from build123d import *

# Parameters (mm, degrees)
SKETCH3_R               = 7.493
CUT_EXTRUDE2_DEPTH      = 8.9375
CUT_EXTRUDE2_DEPTH_BACK = 8.9375
SKETCH4_R               = 11.1125
SKETCH4_R_2             = 26.924
BOSS_EXTRUDE1_DEPTH     = 15.875
BOSS_EXTRUDE2_START     = 22.225
SKETCH7_R               = 6.35
BOSS_EXTRUDE2_DEPTH     = 4.7625
SKETCH5_R               = 2.4257
CUT_EXTRUDE3_DEPTH      = 27.9875
CUT_EXTRUDE3_DEPTH_BACK = 16.8750001


with BuildPart() as part:
    # Sketch1 → Revolve1 (revolve)
    with BuildSketch(Plane(origin=(0, 0, 0), x_dir=(0, 0, -1), z_dir=(1, 0, 0))):
        with BuildLine():
            Line((-20.6375, 0), (-26.9875, 0))
            Line((-26.9875, 0), (-26.9875, 7.9375))
            Line((-26.9875, 7.9375), (-25.587155577, 7.9375))
            ThreePointArc((-25.587155577, 7.9375), (-23.1775, 5.6515), (-20.767844423, 7.9375))
            Line((-20.767844423, 7.9375), (-19.3675, 7.9375))
            Line((-19.3675, 7.9375), (-19.3675, 5.495734842))
            Line((-19.3675, 5.495734842), (-20.6375, 4.7625))
            Line((-20.6375, 4.7625), (-20.6375, 0))
        make_face()
    revolve(axis=Axis((0, 0, 0), (0, 1, 0)))

    # Mirror1: part across plane


with BuildPart() as part_1:
    add(part.part)
    add(part.part.mirror(Plane(origin=(0, 0, 20.6375), x_dir=(0, 0, 1), z_dir=(0, 1, 0))))

    # Sketch3 → Cut-Extrude2 (cut, two sides)
    with BuildSketch(Plane(origin=(0, 0, 0), x_dir=(1, 0, 0), z_dir=(0, 1, 0))) as cut_extrude2_sk:
        with Locations((12.7, 0)):
            Circle(SKETCH3_R)
    extrude(amount=CUT_EXTRUDE2_DEPTH, mode=Mode.SUBTRACT)
    extrude(cut_extrude2_sk.sketch, amount=-CUT_EXTRUDE2_DEPTH_BACK, mode=Mode.SUBTRACT)

    # Sketch4 → Boss-Extrude1 (add, through all)
    with BuildSketch(Plane(origin=(0, 7.9375, 0), x_dir=(1, 0, 0), z_dir=(0, 1, 0))):
        Polygon((28.575, 28.575), (-53.975, 28.575), (-53.975, -12.7), (-12.7, -53.975), (28.575, -53.975), align=None)
        with Locations((-36.890166373, 9.525)):
            Circle(SKETCH4_R, mode=Mode.SUBTRACT)
        with Locations((9.525, -36.890166373)):
            Circle(SKETCH4_R, mode=Mode.SUBTRACT)
        Circle(SKETCH4_R_2, mode=Mode.SUBTRACT)
    extrude(amount=-BOSS_EXTRUDE1_DEPTH)


with BuildPart() as body_2:
    # Sketch7 → Boss-Extrude2 (new body)
    with BuildSketch(Plane(origin=(0, 7.9375, 0), x_dir=(1, 0, 0), z_dir=(0, 1, 0)).offset(BOSS_EXTRUDE2_START)):
        Polygon((28.575, -53.975), (28.575, 28.575), (-53.975, 28.575), (-53.975, -12.7), (-12.7, -53.975), align=None)
        Circle(SKETCH7_R, mode=Mode.SUBTRACT)
    extrude(amount=BOSS_EXTRUDE2_DEPTH)


with BuildPart() as cut_extrude3_tool:
    # Sketch5 → Cut-Extrude3 (new body, two sides)
    with BuildSketch(Plane(origin=(0, 7.9375, 0), x_dir=(1, 0, 0), z_dir=(0, 1, 0))) as cut_extrude3_sk:
        with Locations((23.8125, 23.8125)):
            Circle(SKETCH5_R)
        with Locations((-49.2125, 23.8125)):
            Circle(SKETCH5_R)
        with Locations((-23.933885369, 23.8125)):
            Circle(SKETCH5_R)
        with Locations((-49.2125, -10.727307909)):
            Circle(SKETCH5_R)
        with Locations((23.8125, -23.933885369)):
            Circle(SKETCH5_R)
        with Locations((23.8125, -49.2125)):
            Circle(SKETCH5_R)
        with Locations((-10.727307909, -49.2125)):
            Circle(SKETCH5_R)
    extrude(amount=CUT_EXTRUDE3_DEPTH)
    extrude(cut_extrude3_sk.sketch, amount=-CUT_EXTRUDE3_DEPTH_BACK)


with BuildPart() as part_2:
    add(part_1.part)

    # Cut-Extrude3: cut by cut_extrude3_tool
    add(cut_extrude3_tool.part, mode=Mode.SUBTRACT)


with BuildPart() as body_2_1:
    add(body_2.part)

    # Cut-Extrude3: cut by cut_extrude3_tool
    add(cut_extrude3_tool.part, mode=Mode.SUBTRACT)


solid = part_2.part
Model file for the job. Use its own axes, mm. A direction names the side the tool comes from. Round coordinates to 2 decimals unless told otherwise and drop trailing zeros. Loops run counter-clockwise (first coordinate to the right, second up) from the corner with the lowest first, then second, coordinate; pieces in that order, holes last.
1. Drop a flat-ended pin along its axis: P1, Ø3, axis at x = 23.81, z = -23.81, coming from the -Y side. Give the stop position or say it passes through.
Check values:
P1: passes through
2. Band-saw the part on C-C, the plane x = 0. List the corners of the cut face in (y, z) (1 decimal).
Check values:
outline: (-7.9, -28.6) - (7.9, -28.6) - (7.9, -25.6) arc R2.4 cw to (7.9, -20.8) - (7.9, -19.4) - (5.5, -19.4) - (4.8, -20.6) - (-4.8, -20.6) - (-5.5, -19.4) - (-7.9, -19.4) - (-7.9, -20.8) arc R2.4 cw to (-7.9, -25.6) - close; (-7.9, 19.4) - (-5.5, 19.4) - (-4.8, 20.6) - (4.8, 20.6) - (5.5, 19.4) - (7.9, 19.4) - (7.9, 20.8) arc R2.4 cw to (7.9, 25.6) - (7.9, 31.2) - (-7.9, 31.2) - (-7.9, 25.6) arc R2.4 cw to (-7.9, 20.8) - close; (-7.9, 42.6) - (7.9, 42.6) - (7.9, 54) - (-7.9, 54) - close
3. Wall check: probe 1 along X at (y, z) = (-0.5, 0) (1 decimal); probe 2 along Z at (x, y) = (25.5, 0.5) (3 decimals); probe 3 along Z at (x, y) = (17.5, 0.5) (1 decimal). Give the ranges that are in metal, low to high.
Check values:
probe 1: x = -54 to -42.6, -31.2 to -20.6, 20.6 to 28.6
probe 2: z = -28.575 to -25.555, -22.07 to 22.191, 25.676 to 47.47, 50.955 to 53.975
probe 3: z = -28.6 to -10.9, 10.9 to 29.2, 44.6 to 54
4. Band-saw the part on D-D, the plane x = 22.5. Count the separate pieces of the cut face and the enclosed holes in it, and give its area (3 significant figures).
Check values:
separate pieces: 4
enclosed holes: 0
area: 1,020 mm2
5. Band-saw the part on A-A, the plane x = -29.5. List the corners of the cut face in (y, z) (1 decimal).
Check values:
outline: (-7.9, -28.6) - (7.9, -28.6) - (7.9, -17.8) - (-7.9, -17.8) - close; (-7.9, -1.2) - (7.9, -1.2) - (7.9, 37.2) - (-7.9, 37.2) - close
6. Mould opens along Y. For faces 1 (the cylindrical face through (-46.972, 0.111, 11.656)), 2 (the flat face through (-14, -7.938, 14)), 3 (the cylindrical face through (-20.147, -0.067, -4.474)) say: +Y half, -Y half, draft (parallel to the pull), parting line (faces both ways), or undercut.
Check values:
face 1: draft
face 2: -Y half
face 3: undercut
7. Tool access for faces 4 (the flat face through (-12, 0, -28.575)), 5 (the conical face through (-17.378, 5.368, 9.039)), 6 (the cylindrical face through (20.193, -6.458, 0.062)): list every direction of +Z, -Z, +X, -X, +Y, -Y with a clear straight run to the whole face (end or side of a thin tool).
Check values:
face 4: -Z, +X, -X, +Y, -Y
face 5: none
face 6: +Y, -Y
8. Band-saw the part on B-B, the plane z = 0. List the corners of the cut face in (x, y) (1 decimal), and give its area (3 significant figures).
Check values:
outline: (-54, -7.9) - (-42.6, -7.9) - (-42.6, 7.9) - (-54, 7.9) - close; (-31.2, -7.9) - (-25.6, -7.9) arc R2.4 cw to (-20.8, -7.9) - (-19.4, -7.9) - (-19.4, -5.5) - (-20.6, -4.8) - (-20.6, 4.8) - (-19.4, 5.5) - (-19.4, 7.9) - (-20.8, 7.9) arc R2.4 cw to (-25.6, 7.9) - (-31.2, 7.9) - close; (20.2, -7.9) - (20.8, -7.9) arc R2.4 cw to (25.6, -7.9) - (28.6, -7.9) - (28.6, 7.9) - (25.6, 7.9) arc R2.4 cw to (20.8, 7.9) - (20.2, 7.9) - (20.2, 5) - (20.6, 4.8) - (20.6, -4.8) - (20.2, -5) - close
area: 449 mm2
